from build123d import *

# Parameters (mm, degrees)
F2_R    = 0.4
F3_SIZE = 0.3


with BuildPart() as f1:
    # F0 (on Right) → F1 (revolve)
    with BuildSketch(Plane.YZ):
        Polygon((0, 5.5), (0, 2.55), (16.554633, 2.55), (16.554633, 3.8), (10, 3.8), (7, 4.2), (5.5, 4.2), (5, 3.9), (3, 3.9), (3, 5.5), align=None)
    revolve(axis=Axis((0, 9.707107, 0), (0, 1, 0)))

    # F2
    f2_edges = [f1.edges().sort_by_distance(p)[0] for p in [
        (0, 3, -3.9),
    ]]
    fillet(f2_edges, radius=F2_R)

    # F3
    f3_edges = [f1.edges().sort_by_distance(p)[0] for p in [
        (0, 3, -5.5),
        (0, 0, -5.5),
        (0, 16.554633, -3.8),
        (0, 0, -2.55),
    ]]
    chamfer(f3_edges, length=F3_SIZE)


solid = f1.part
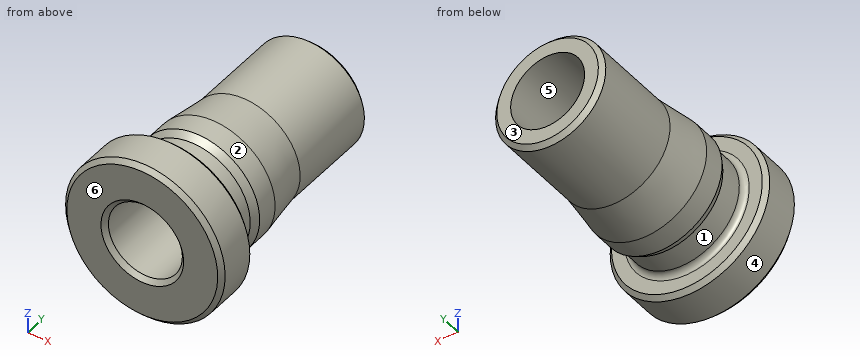
Can you work these out from the model? Positions are in its coordinate system, mm. Face numbers are marked on the shaded views. A direction names the side the tool comes from. Give positions to 0.01 mm unless a question says otherwise; leave off trailing zeros. Order: outer loops, then holes, each group sorted by start corner. A loop starts at its lowest first (then second) coordinate and runs counter-clockwise, first axis right, second up. Notation, with made-up numbers: (65, 37) - (124, 37) arc R33 cw to (124, 67) - close; hole circle Ø4 at (-29.5, 13.5). An arc over 180 degrees is marked (long way). Write each question's results on one line, items separated by ' | '.
1) On a 3-axis mill with a long thin cutter (end or side, diameter ignored), from which of +Z, -Z, +X, -X, +Y, -Y can I reach the whole of each face in a straight line? I mean the marked faces 1, 2 and 3. Say none if no direction works.
Final values:
face 1: none | face 2: +Y | face 3: +Z, -Z, +X, -X, +Y
2) If we mould it in two halves opening along Z, with no side actions, what happens to the marked faces 4, 5 and 6? For each: pulls with the +Z half, pulls with the -Z half, needs draft (parallel to the pull), parting line crosses it, or undercut.
Final values:
face 4: parting line crosses it | face 5: undercut | face 6: needs draft
3) Please list where these lines run through material, in increasing order: line 1 along X through (y, z) = (10, 0); line 2 along X through (y, z) = (4, 0); line 3 along Y through (x, z) = (-4.5, -0.25). Write a range as [from, to].
Final values:
line 1: x = [-3.8, -2.55], [2.55, 3.8] | line 2: x = [-3.9, -2.55], [2.55, 3.9] | line 3: y = [0, 3]
4) Suppose I cut it at C-C, the plane y = 13.75. Write out the boundary of the cut face in (x, z).
Final values:
outline: circle Ø7.6 at (0, 0); hole circle Ø5.1 at (0, 0)
5) Suppose I cut it at D-D, the plane y = 5.75. Write out the boundary of the cut face in (x, z).
Final values:
outline: circle Ø8.4 at (0, 0); hole circle Ø5.1 at (0, 0)
6) I'm going to push flat-ended pins straight in: pin 1 Ø2 at (x, y) = (4, 11.5) entering from -Z; pin 2 Ø2 at (x, z) = (-2, -4) entering from -Y. Where does each tip first touch, or does it pass through?
Final values:
pin 1: stops at z = -2.33 | pin 2: stops at y = 0
